Could you check a few things on this model? Use its own coordinates, in mm. Face numbers are marked on the shaded views. A direction names the side the tool comes from. Coordinates: 2 decimals unless noted, no trailing zeros. Use a Markdown table: item, result. Add a question column.
1) Which directions (+Z, -Z, +X, -X, +Y, -Y) give clear straight access to the entire face, cutting with the end or side of a thin tool? Please do the marked faces 1 and 2.
2) Thinking about a two-plate mould opening in X: for the marked faces 3, 4, 5 and 6, which applies, +X half, -X half, draft (parallel to the pull), parting line (faces both ways), or undercut?
3) If I drill on L1, parallel to X at y = 0, z = 30.5 (1 decimal); L2, parallel to X at y = 6, z = 12; L3, parallel to Y at x = 0, z = 25 (1 decimal), over which ranges is the centre line in solid material (lowest first)? Write a range as [from, to].
4) If we section it at A-A (z = 13.5): Give the number of separate pieces and of enclosed holes in the cut face, plus the area to 3 significant figures.
5) Will these pins go through, and if not, where does the flat tip stop? pin 1 Ø1 at (x, z) = (23, 5.5) entering from -Y; pin 2 Ø8 at (y, z) = (-15.5, 25) entering from +X; pin 3 Ø3 at (y, z) = (15, 6) entering from -X.
```python
from build123d import *

# Parameters (mm, degrees)
F1_DEPTH = 40.2336
F2_DEPTH = 15.7734
F3_R     = 3.302


with BuildPart() as f1:
    # F0 (on Top) → F1 (new body)
    with BuildSketch(Plane.XY):
        with BuildLine():
            ThreePointArc((9.738373, -26.864376), (23.39663, -16.405131), (28.575, 0))
            ThreePointArc((28.575, 0), (23.327466, 16.503332), (9.512184, 26.945296))
            ThreePointArc((9.512184, 26.945296), (-28.574748, -0.120114), (9.738373, -26.864376))
        make_face()
        with BuildLine():
            Line((18.5293, 4.826), (18.5293, 0))
            Line((18.5293, 0), (18.5293, -4.826))
            Line((18.5293, -4.826), (13.447765, -4.826))
            ThreePointArc((13.447765, -4.826), (-14.2875, 0), (13.447765, 4.826))
            Line((13.447765, 4.826), (18.5293, 4.826))
        make_face(mode=Mode.SUBTRACT)
    extrude(amount=F1_DEPTH)

    # F0 (on Top) → F2 (join)
    with BuildSketch(Plane.XY):
        with BuildLine():
            ThreePointArc((9.512184, 26.945296), (23.327466, 16.503332), (28.575, 0))
            ThreePointArc((28.575, 0), (23.39663, -16.405131), (9.738373, -26.864376))
            Line((9.738373, -26.864376), (54.234754, -19.048229))
            ThreePointArc((54.234754, -19.048229), (72.967046, -1.48482), (57.191927, 18.776418))
            Line((57.191927, 18.776418), (9.512184, 26.945296))
        make_face()
        with BuildLine():
            ThreePointArc((64.135, 0), (53.975, -10.16), (43.815, 0))
            ThreePointArc((43.815, 0), (53.975, 10.16), (64.135, 0))
        make_face(mode=Mode.SUBTRACT)
    extrude(amount=F2_DEPTH)

    # F3
    f3_edges = [f1.edges().sort_by_distance(p)[0] for p in [
        (-9.738373, 26.864376, 40.2336),
    ]]
    fillet(f3_edges, radius=F3_R)


solid = f1.part
```
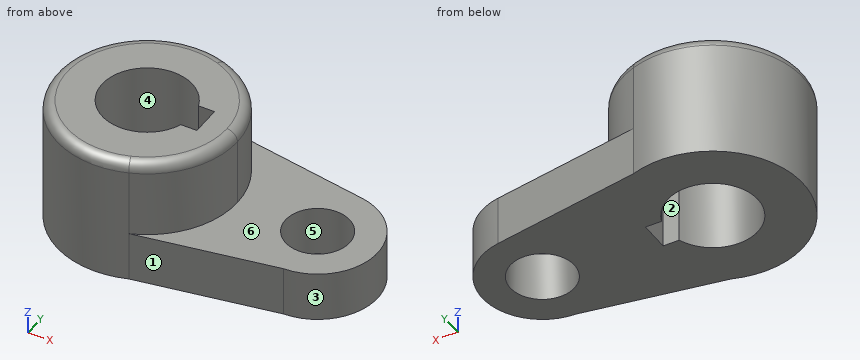
Answer sheet:
| question | item | result |
|---|---|---|
| 1 | face 1 | +Z, -Z, +X, -Y |
| 1 | face 2 | +Z, -Z |
| 2 | face 3 | +X half |
| 2 | face 4 | undercut |
| 2 | face 5 | undercut |
| 2 | face 6 | draft |
| 3 | L1 | [-28.6, -14.3], [18.5, 28.6] |
| 3 | L2 | [-27.94, -12.97], [12.97, 45.78], [62.17, 72.06] |
| 3 | L3 | [-28.6, -14.3], [14.3, 28.6] |
| 4 | separate pieces | 1 |
| 4 | enclosed holes | 2 |
| 4 | area | 3,430 mm2 |
| 5 | pin 1 | y = -24.62 |
| 5 | pin 2 | x = 26.16 |
| 5 | pin 3 | x = -25.18 |
